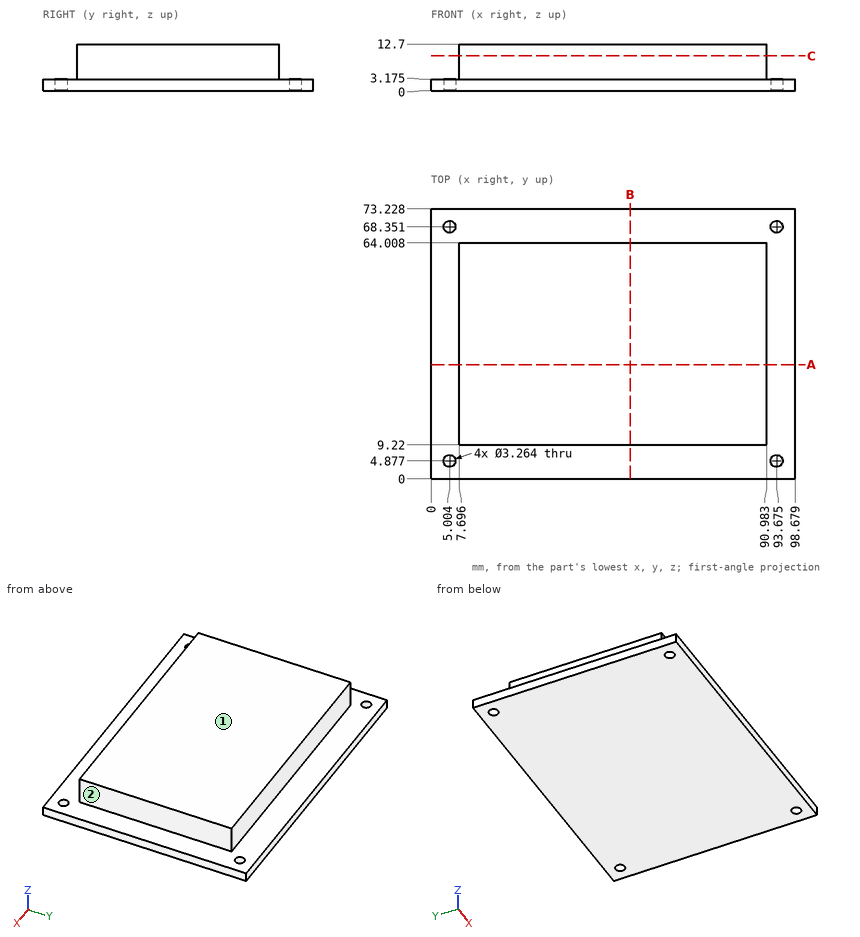
Input: dimensioned drawing with shaded views. Units: mm. Origin: part minimum x, y, z. A direction names the side the tool comes from. Give positions to 0.01 mm unless a question says otherwise; leave off trailing zeros. Loops run counter-clockwise (first coordinate to the right, second up) from the corner with the lowest first, then second, coordinate; pieces in that order, holes last. Notation, with made-up numbers: (-33.75, 0.5) - (-8.75, 0.5) arc R26 ccw to (-8.75, 21.5) - close; hole circle Ø10 at (-4.75, 68). An arc over 180 degrees is marked (long way). Answer as CSV lines item,"result". Start each with the question number.
(1) Section query A-A (y = 31). Output: boundary loops of the cut face in (x, z) (1 decimal).
(2) Ray query, line 1 along X through (y, z) = (62, 5.25); line 2 along Y through (x, z) = (59.5, 8.5); line 3 along Z through (x, y) = (19, 65.5) (1 decimal). Return the intervals inside material, ascending. Write a range as [from, to].
(3) Reachability of the marked faces 1 and 2 from +Z, -Z, +X, -X, +Y, -Y: full face, straight path, thin tool, end or side. Return the list, or none.
(4) Section query B-B (x = 54). Output: boundary loops of the cut face in (y, z) (1 decimal).
(5) Section query C-C (z = 9.5). Output: boundary loops of the cut face in (x, y).
(6) Pin query (flat end, axial travel): P1, Ø5, axis at x = 5, y = 68.35, coming from the +Z side (3 decimals); P2, Ø3, axis at x = 36.5, z = 8, coming from the +Y side; P3, Ø3, axis at x = 5, y = 4.88, coming from the +Z side; P4, Ø7.5, axis at y = 48.5, z = 7, coming from the -X side. Return the tip coordinate at first contact, or that it passes through.
Worked answers:
1,outline,"(0, 0) - (98.7, 0) - (98.7, 3.2) - (91, 3.2) - (91, 12.7) - (7.7, 12.7) - (7.7, 3.2) - (0, 3.2) - close"
2,line 1,"x = [7.7, 90.98]"
2,line 2,"y = [9.22, 64.01]"
2,line 3,"z = [0, 3.2]"
3,face 1,"+Z, +X, -X, +Y, -Y"
3,face 2,"+Z, +X, +Y, -Y"
4,outline,"(0, 0) - (73.2, 0) - (73.2, 3.2) - (64, 3.2) - (64, 12.7) - (9.2, 12.7) - (9.2, 3.2) - (0, 3.2) - close"
5,outline,"(7.7, 9.22) - (90.98, 9.22) - (90.98, 64.01) - (7.7, 64.01) - close"
6,P1,"stops at z = 3.175"
6,P2,"stops at y = 64.01"
6,P3,"passes through"
6,P4,"stops at x = 7.7"
